Read the model definition and answer for the solid it produces. Units are mm, in the model's axes. Face numbers are marked on the shaded views. A direction names the side the tool comes from. Round coordinates to 2 decimals unless told otherwise and drop trailing zeros. Write each loop counter-clockwise with the first axis right and the second up, starting at its lowest first coordinate (ties: lowest second). Pieces come first, ordered by that corner, then holes. Notation, with made-up numbers: (77.25, 89) - (129.25, 89) arc R14 cw to (129.25, 95) - close; hole circle Ø9 at (84, -28). An arc over 180 degrees is marked (long way). One line per item, written item: value. Start each with the question number.
(1) For the marked faces 1, 2 and 3, determine the directions among +Z, -Z, +X, -X, +Y, -Y from which every point of the face is accessible in a straight line to the end or side of a thin tool.
(2) Find the intervals of material crossed by L1, parallel to Z at x = 23, y = -114.3 (3 decimals); L2, parallel to X at y = -40, z = -0.5; L3, parallel to Z at x = 4, y = -86.5, in increasing order.
(3) Flat-ended cylindrical pins translate along their axes: pin 1 Ø6 at (x, z) = (20.5, 4) entering from -Y; pin 2 Ø4 at (y, z) = (-55.5, -3.5) entering from -X; pin 3 Ø4 at (y, z) = (-13.5, 3.5) entering from +X. Find the tip coordinate at first contact, or state that the pin passes through.
(4) A cutting plane is placed at C-C, the plane y = -76. Determine the outline of the cut face in (x, z).
(5) A cutting plane is placed at A-A, the plane z = 0. Determine the outline of the cut face in (x, y) (3 decimals), plus the area to 3 significant figures.
(6) A cutting plane is placed at B-B, the plane x = 17.5. Determine the outline of the cut face in (y, z), plus the area to 3 significant figures.
from build123d import *

# Parameters (mm, degrees)
SKETCH1_R          = 6.35
SKETCH3_R          = 3.175
CUT_EXTRUDE1_DEPTH = 6.35


with BuildPart() as part:
    # Sweep1: sweep along a path in Sketch2
    with BuildLine(Plane.XY) as sweep1_path:
        Line((0, 0), (0, -101.6))
        ThreePointArc((0, -101.6), (3.719743879, -110.580256121), (12.7, -114.3))
        Line((12.7, -114.3), (25.4, -114.3))
    # Sketch1 → Sweep1 (sweep)
    with BuildSketch(Plane(origin=(0, 0, 0), x_dir=(1, 0, 0), z_dir=(0, 1, 0))):
        Circle(SKETCH1_R)
    sweep(path=sweep1_path.line)

    # Sketch3 → Cut-Extrude1 (cut)
    with BuildSketch(Plane(origin=(25.4, 0, 0), x_dir=(0, 0, -1), z_dir=(1, 0, 0))):
        with Locations(Location((0, -114.3, 0), (0, 0, 90))):
            Circle(SKETCH3_R)
    extrude(amount=-CUT_EXTRUDE1_DEPTH, mode=Mode.SUBTRACT)


solid = part.part
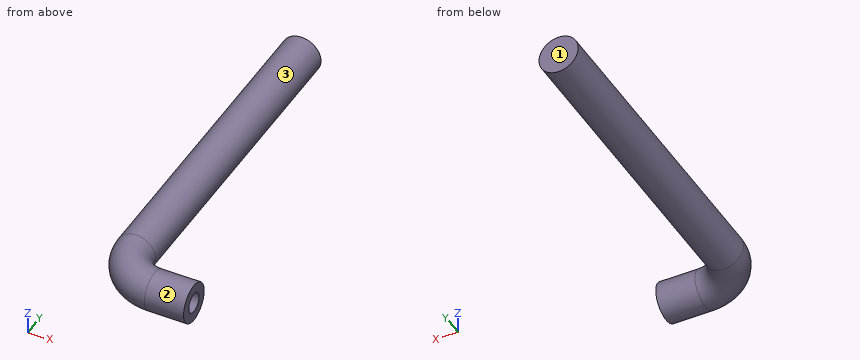
Here are the results:
1. face 1: +Z, -Z, +X, -X, +Y
1. face 2: +X
1. face 3: +Y
2. L1: -6.35 to -3.175, 3.175 to 6.35
2. L2: -6.33 to 6.33
2. L3: -4.93 to 4.93
3. pin 1: y = -120.57
3. pin 2: x = -6.17
3. pin 3: x = 6.17
4. outline: circle Ø12.7 at (0, 0)
5. outline: (-6.35, -101.6) arc R19.05 ccw to (12.7, -120.65) - (25.4, -120.65) - (25.4, -117.475) - (19.05, -117.475) - (19.05, -111.125) - (25.4, -111.125) - (25.4, -107.95) - (12.7, -107.95) arc R6.35 cw to (6.35, -101.6) - (6.35, 0) - (-6.35, 0) - close
5. area: 1,660 mm²
6. outline: circle Ø12.7 at (-114.3, 0)
6. area: 127 mm²
